Autodesk Inventor part; units mm, degrees
ref_plane "YZ Plane" through (0, 0, 0) normal (1, 0, 0) x (0, 1, 0)
ref_plane "XZ Plane" through (0, 0, 0) normal (0, 1, 0) x (-1, 0, 0)
ref_plane "XY Plane" through (0, 0, 0) normal (0, 0, 1) x (1, 0, 0)
sketch "Sketch1" plane through (0, 0, 0) normal (0, 0, 1) x (1, 0, 0)
  circle A0 centre (0, 0) radius 2
  dimension "Diameter" = 4
extrude "Extrusion1" add sketch "Sketch1" along normal blind 17.52
sketch "Sketch2" plane through (0, 0, 17.52) normal (0, 0, 1) x (1, 0, 0)
  circle A0 centre (0, 0) radius 2
extrude "Extrusion2" add sketch "Sketch2" along normal blind 2.48 draft 45
sketch "Sketch3" plane through (0, 0, 20) normal (0, 0, 1) x (1, 0, 0)
  circle A0 centre (0, 0) radius 4.48
  circle A1 centre (0, 0) radius 1.4434 construction
  line L0 (0.6042, 1.3108) -> (1.4373, 0.1322)
  line L1 (1.4373, 0.1322) -> (0.8331, -1.1787)
  line L2 (0.8331, -1.1787) -> (-0.6042, -1.3108)
  line L3 (-0.6042, -1.3108) -> (-1.4373, -0.1322)
  line L4 (-1.4373, -0.1322) -> (-0.8331, 1.1787)
  line L5 (-0.8331, 1.1787) -> (0.6042, 1.3108)
  dimension "Hex_Width" = 2.5
extrude "Extrusion3" cut sketch "Sketch3" against normal blind 1.5 contours L0 L1 L2 L3 L4 L5
thread "Thread1"
chamfer "Chamfer2" distance 0.4 angle 45 1 edges at (-2, 0, 0)
fillet "Fillet1" radius 0.1 1 edges at (-4.48, 0, 20)
equation "\"d13\" = Chamfer"
equation "\"Thread_Length\" = 7.52"
properties part number "SCREW, FLAT HD, P, 12_9, M4X0_7X20"
Read the model definition and answer for the solid it produces. Units are mm, in the model's axes. A direction names the side the tool comes from. Round coordinates to 2 decimals unless told otherwise and drop trailing zeros. Write each loop counter-clockwise with the first axis right and the second up, starting at its lowest first coordinate (ties: lowest second). Pieces come first, ordered by that corner, then holes. Notation, with made-up numbers: (70.25, 32) -> (111.25, 32) arc R9 ccw to (111.25, 45) -> close; hole circle Ø4 at (26.25, 58.25). An arc over 180 degrees is marked (long way). Answer in a Markdown table with one row per item. Add a question column.
1) Consider line 1 (X direction, y = 0, z = 12.5); line 2 (Z direction, x = 0.5, y = 0.5); line 3 (Z direction, x = 1, y = 2.5). Determine where each line is inside the solid, lowest interval first.
2) Find section C-C, the plane z = 10.75. Determine the outline of the cut face in (x, y), and give its area (3 significant figures).
3) Determine the mould class of faces 1 (the face through (2.045, 0.644, 17.664)), 2 (the face through (-0.125, 1.244, 19.26)), 3 (the face through (0, -2, 20)) for opening direction X: pulls with the +X half, pulls with the -X half, needs draft (parallel to the pull), parting line crosses it, or undercut.
4) Given P1, Ø2, axis at x = 1, z = 6.5, coming from the -Y side; P2, Ø5, axis at x = 1.5, z = 17.5, coming from the +Y side; P3, Ø5, axis at x = -0.5, z = 11, coming from the +Y side, each flat-ended and moving along its own axis, determine where each tip first touches the part or whether it passes through.
5) Which of the six approach directions +Z, -Z, +X, -X, +Y, -Y give full straight-line access (tool end or side, diameter ignored) to faces 4 (the face through (0, 0, 0)), 5 (the face through (0, 0, 18.5)), 6 (the face through (0, 2, 9))?
6) Find section A-A, the plane z = 18.75. Determine the outline of the cut face in (x, y).
7) Find section B-B, the plane x = 0. Determine the outline of the cut face in (y, z), and give its area (3 significant figures).
Findings below:
| question | item | result |
|---|---|---|
| 1 | line 1 | -2 to 2 |
| 1 | line 2 | 0 to 18.5 |
| 1 | line 3 | 18.21 to 20 |
| 2 | outline | circle Ø4 at (0, 0) |
| 2 | area | 12.6 mm² |
| 3 | face 1 | parting line crosses it |
| 3 | face 2 | undercut |
| 3 | face 3 | needs draft |
| 4 | P1 | y = -2 |
| 4 | P2 | y = 4.28 |
| 4 | P3 | y = 2 |
| 5 | face 4 | -Z, +X, -X, +Y, -Y |
| 5 | face 5 | +Z |
| 5 | face 6 | -Z |
| 6 | outline | circle Ø6.46 at (0, 0); hole (-1.44, -0.13) -> (-0.6, -1.31) -> (0.83, -1.18) -> (1.44, 0.13) -> (0.6, 1.31) -> (-0.83, 1.18) -> close |
| 7 | outline | (-4.31, 19.83) -> (-2, 17.52) -> (-2, 0.4) -> (-1.6, 0) -> (1.6, 0) -> (2, 0.4) -> (2, 17.52) -> (4.31, 19.83) arc R0.1 ccw to (4.24, 20) -> (1.26, 20) -> (1.26, 18.5) -> (-1.26, 18.5) -> (-1.26, 20) -> (-4.24, 20) arc R0.1 ccw to start |
| 7 | area | 82.2 mm² |
